Verification items for the finished model (mm, model axes). A direction names the side the tool comes from. Give positions to 0.01 mm unless a question says otherwise; leave off trailing zeros. Order: outer loops, then holes, each group sorted by start corner. A loop starts at its lowest first (then second) coordinate and runs counter-clockwise, first axis right, second up.
from build123d import *

# Parameters (mm, degrees)
SKETCH1_W           = 35
SKETCH1_H           = 31
BOSS_EXTRUDE1_DEPTH = 15
CUT_EXTRUDE1_DEPTH  = 4
SKETCH3_W           = 35
SKETCH3_H           = 15
BOSS_EXTRUDE2_DEPTH = 4
SKETCH4_W           = 11
SKETCH4_H           = 31
CUT_EXTRUDE2_DEPTH  = 31
CUT_EXTRUDE3_DEPTH  = 48.021271782
CUT_EXTRUDE4_DEPTH  = 54.018864567
CUT_EXTRUDE5_DEPTH  = 54.018864567
CUT_EXTRUDE6_DEPTH  = 50.749371855


with BuildPart() as part:
    # Sketch1 → Boss-Extrude1 (new body)
    with BuildSketch(Plane(origin=(0, 0, 10), x_dir=(-1, 0, 0), z_dir=(0, 0, -1))):
        with Locations((-7.5, -19.5)):
            Rectangle(SKETCH1_W, SKETCH1_H)
    extrude(amount=-BOSS_EXTRUDE1_DEPTH)

    # Sketch2 → Cut-Extrude1 (cut)
    with BuildSketch(Plane(origin=(0, 0, 10), x_dir=(-1, 0, 0), z_dir=(0, 0, -1))):
        Polygon((10, -4), (-21, -35), (10, -35), align=None)
    extrude(amount=-CUT_EXTRUDE1_DEPTH, mode=Mode.SUBTRACT)

    # Sketch3 → Boss-Extrude2 (add)
    with BuildSketch(Plane(origin=(0, -4, 0), x_dir=(-1, 0, 0), z_dir=(0, 1, 0))):
        with Locations((-7.5, 17.5)):
            Rectangle(SKETCH3_W, SKETCH3_H)
    extrude(amount=BOSS_EXTRUDE2_DEPTH)

    # Sketch4 → Cut-Extrude2 (cut)
    with BuildSketch(Plane.ZY.offset(10)):
        with Locations((19.5, -19.5)):
            Rectangle(SKETCH4_W, SKETCH4_H)
    extrude(amount=-CUT_EXTRUDE2_DEPTH, mode=Mode.SUBTRACT)

    # Sketch5 → Cut-Extrude3 (cut, through all)
    with BuildSketch(Plane.XZ.offset(4)):
        Polygon((-2.75, 16.20096), (-2.388229, 16.05111), (-2, 16), (-1.611771, 16.05111), (-1.25, 16.20096), (-0.9393398, 16.43934), (-0.7009619, 16.75), (-0.5511113, 17.11177), (-0.5, 17.5), (-0.5511113, 17.88823), (-0.7009619, 18.25), (-0.9393398, 18.56066), (-1.25, 18.79904), (-1.611771, 18.94889), (-2, 19), (-2.388229, 18.94889), (-2.75, 18.79904), (-3.06066, 18.56066), (-3.299038, 18.25), (-3.448889, 17.88823), (-3.5, 17.5), (-3.448889, 17.11177), (-3.299038, 16.75), (-3.06066, 16.43934), align=None)
    extrude(amount=-CUT_EXTRUDE3_DEPTH, mode=Mode.SUBTRACT)

    # Sketch6 → Cut-Extrude4 (cut, through all)
    with BuildSketch(Plane.ZY.offset(-21)):
        Polygon((17.11177, -28.44889), (17.5, -28.5), (17.88823, -28.44889), (18.25, -28.29904), (18.56066, -28.06066), (18.79904, -27.75), (18.94889, -27.38823), (19, -27), (18.94889, -26.61177), (18.79904, -26.25), (18.56066, -25.93934), (18.25, -25.70096), (17.88823, -25.55111), (17.5, -25.5), (17.11177, -25.55111), (16.75, -25.70096), (16.43934, -25.93934), (16.20096, -26.25), (16.05111, -26.61177), (16, -27), (16.05111, -27.38823), (16.20096, -27.75), (16.43934, -28.06066), (16.75, -28.29904), align=None)
    extrude(amount=-CUT_EXTRUDE4_DEPTH, mode=Mode.SUBTRACT)

    # Sketch7 → Cut-Extrude5 (cut, through all)
    with BuildSketch(Plane.ZY.offset(-21)):
        Polygon((16.20096, -11.75), (16.43934, -12.06066), (16.75, -12.29904), (17.11177, -12.44889), (17.5, -12.5), (17.88823, -12.44889), (18.25, -12.29904), (18.56066, -12.06066), (18.79904, -11.75), (18.94889, -11.38823), (19, -11), (18.94889, -10.61177), (18.79904, -10.25), (18.56066, -9.93934), (18.25, -9.700962), (17.88823, -9.551111), (17.5, -9.5), (17.11177, -9.551111), (16.75, -9.700962), (16.43934, -9.93934), (16.20096, -10.25), (16.05111, -10.61177), (16, -11), (16.05111, -11.38823), align=None)
    extrude(amount=-CUT_EXTRUDE5_DEPTH, mode=Mode.SUBTRACT)

    # Sketch8 → Cut-Extrude6 (cut, through all)
    with BuildSketch(Plane(origin=(0, 0, 0), x_dir=(-1, 0, 0), z_dir=(0, 1, 0))):
        Polygon((-12.70096, 16.75), (-12.55111, 17.11177), (-12.5, 17.5), (-12.55111, 17.88823), (-12.70096, 18.25), (-12.93934, 18.56066), (-13.25, 18.79904), (-13.61177, 18.94889), (-14, 19), (-14.38823, 18.94889), (-14.75, 18.79904), (-15.06066, 18.56066), (-15.29904, 18.25), (-15.44889, 17.88823), (-15.5, 17.5), (-15.44889, 17.11177), (-15.29904, 16.75), (-15.06066, 16.43934), (-14.75, 16.20096), (-14.38823, 16.05111), (-14, 16), (-13.61177, 16.05111), (-13.25, 16.20096), (-12.93934, 16.43934), align=None)
    extrude(amount=-CUT_EXTRUDE6_DEPTH, mode=Mode.SUBTRACT)


solid = part.part
(1) Section check A-A, the plane z = 23.5. Enter the section's corners in (x, y).
Solved:
outline: (-10, -4) - (21, -4) - (21, -35) - (25, -35) - (25, 0) - (-10, 0) - close
(2) Go/stop test with flat-tipped pins: pin 1 (5 mm diameter, centred on x = 15, y = -8.5, fed in from +Z); pin 2 (5 mm diameter, centred on x = 1, y = -4.5, fed in from +Z); pin 3 (5 mm diameter, centred on x = 14.5, z = 21.5, fed in from -Y). Record where each tip stops, or that it passes through.
Solved:
pin 1: stops at z = 14
pin 2: stops at z = 25
pin 3: stops at y = -4
(3) Set-up check for faces 1 (the flat face through (23, -35, 17)), 2 (the flat face through (5, -4, 19)): record each of +Z, -Z, +X, -X, +Y, -Y from which the full face is reachable in a straight line by a thin tool's end or side.
Solved:
face 1: +Z, -Z, +X, -X, -Y
face 2: +Z, -X, -Y
(4) Section check C-C, the plane x = 21.5. Give the number of separate pieces and of enclosed holes in the cut face, then the cut area to 3 significant figures.
Solved:
separate pieces: 1
enclosed holes: 2
area: 511 mm2
(5) Scan lines: line 1 (Y direction, x = 14, z = 20.5); line 2 (X direction, y = -5.5, z = 20.5); line 3 (Z direction, x = -2.5, y = -6). Record each from-to range of solid material in increasing order.
Solved:
line 1: y = -4 to 0
line 2: x = 21 to 25
line 3: z = 10 to 14
(6) Section check D-D, the plane z = 11.25. Enter the section's corners in (x, y), then the cut area to 4 significant figures.
Solved:
outline: (-10, -4) - (21, -35) - (25, -35) - (25, 0) - (-10, 0) - close
area: 744.5 mm2
(7) Section check B-B, the plane x = 2.5. Enter the section's corners in (y, z), then the cut area to 3 significant figures.
Solved:
outline: (-16.5, 10) - (0, 10) - (0, 25) - (-4, 25) - (-4, 14) - (-16.5, 14) - close
area: 110 mm2
